```python
from build123d import *

# Parameters (mm, degrees)
BOSS_EXTRUDE1_DEPTH = 84.666666667
SKETCH2_R           = 53.34
CUT_EXTRUDE1_DEPTH  = 85.666666667
SKETCH3_W           = 25.4
SKETCH3_H           = 25.4
BOSS_EXTRUDE2_DEPTH = 44.45
SKETCH5_R           = 3.175
CUT_EXTRUDE2_DEPTH  = 70.215


with BuildPart() as part:
    # Sketch1 → Boss-Extrude1 (new body)
    with BuildSketch(Plane.XY):
        with BuildLine():
            Line((-12.7, -56.515), (12.7, -56.515))
            Line((12.7, -56.515), (12.7, -55.069548981))
            ThreePointArc((12.7, -55.069548981), (0, 56.515), (-12.7, -55.069548981))
            Line((-12.7, -55.069548981), (-12.7, -56.515))
        make_face()
    extrude(amount=BOSS_EXTRUDE1_DEPTH)

    # Sketch2 → Cut-Extrude1 (cut, through all)
    with BuildSketch(Plane.XY.offset(84.666666667)):
        Circle(SKETCH2_R)
    extrude(amount=-CUT_EXTRUDE1_DEPTH, mode=Mode.SUBTRACT)

    # Sketch3 → Boss-Extrude2 (add)
    with BuildSketch(Plane.XZ.offset(56.515)):
        with Locations((0, 42.333333333)):
            Rectangle(SKETCH3_W, SKETCH3_H)
    extrude(amount=BOSS_EXTRUDE2_DEPTH)

    # Sketch5 → Cut-Extrude2 (cut, through all)
    with BuildSketch(Plane(origin=(12.7, 0, 0), x_dir=(0, 0, -1), z_dir=(1, 0, 0))):
        with Locations((-42.333333333, -75.565)):
            Circle(SKETCH5_R)
    extrude(amount=-CUT_EXTRUDE2_DEPTH, mode=Mode.SUBTRACT)


solid = part.part
```
For this review, take the finished solid that the model builds, in its own axes (mm). A direction names the side the tool comes from. Coordinates: 2 decimals unless noted, no trailing zeros. Write each loop counter-clockwise with the first axis right and the second up, starting at its lowest first coordinate (ties: lowest second). Pieces come first, ordered by that corner, then holes.
(1) Add section C-C on x = 0. Give the boundary of the cut face in (y, z) (3 decimals).
(2) Tool access review of faces 1 (the face through (0, -56.515, 15)), 2 (the face through (-12.7, -73, 45)), 3 (the face through (12.7, -78, 45)), 4 (the face through (0, -78, 55.033)): name each direction out of +Z, -Z, +X, -X, +Y, -Y from which nothing blocks a thin tool from reaching the whole face with its end or side.
(3) Add section A-A on y = 0. Give the boundary of the cut face in (x, z) (3 decimals).
(4) The part is to be moulded in two halves that separate along Y. For faces 5 (the face through (0.178, -75.425, 45.505)), 6 (the face through (-6.944, 52.886, 42.926)), 7 (the face through (0, -78, 29.633)), 8 (the face through (0, -56.515, 70)), say which applies: +Y half, -Y half, draft (parallel to the pull), parting line (faces both ways), or undercut.
(5) Wall thickness on probe 1 along Y at (x, z) = (0, 42) (3 decimals); probe 2 along Y at (x, z) = (-2, 21) (1 decimal); probe 3 along X at (y, z) = (-1, 15.5): over which ranges is each line inside the solid? List them lowest first.
(6) For pin 1 Ø23 at (y, z) = (-68.5, 40.5) entering from +X; pin 2 Ø7.5 at (x, y) = (4.5, -83) entering from -Z; pin 3 Ø20.5 at (x, z) = (3.5, 71) entering from -Y (3 decimals), all flat-tipped, find the tip position at first contact; note any pin that passes through.
(7) Add section D-D on x = 28.5. Give the boundary of the cut face in (y, z).
(8) Add section B-B on z = 8. Give the boundary of the cut face in (x, y) (3 decimals), then the cut area to 3 significant figures.
Answer sheet:
1. outline: (-100.965, 29.633) - (-56.515, 29.633) - (-56.515, 0) - (-53.34, 0) - (-53.34, 84.667) - (-56.515, 84.667) - (-56.515, 55.033) - (-100.965, 55.033) - close; (53.34, 0) - (56.515, 0) - (56.515, 84.667) - (53.34, 84.667) - close; hole circle Ø6.35 at (-75.565, 42.333)
2. face 1: -Z, +X, -X, -Y
2. face 2: +Z, -Z, -X, -Y
2. face 3: +Z, -Z, +X, -Y
2. face 4: +Z, +X, -X, -Y
3. outline: (-56.515, 0) - (-53.34, 0) - (-53.34, 84.667) - (-56.515, 84.667) - close; (53.34, 0) - (56.515, 0) - (56.515, 84.667) - (53.34, 84.667) - close
4. face 5: undercut
4. face 6: undercut
4. face 7: draft
4. face 8: -Y half
5. probe 1: y = -100.965 to -78.722, -72.408 to -53.34, 53.34 to 56.515
5. probe 2: y = -56.5 to -53.3, 53.3 to 56.5
5. probe 3: x = -56.51 to -53.33, 53.33 to 56.51
6. pin 1: stops at x = 12.7
6. pin 2: stops at z = 29.63
6. pin 3: stops at y = -56.515
7. outline: (-48.8, 0) - (-45.09, 0) - (-45.09, 84.67) - (-48.8, 84.67) - close; (45.09, 0) - (48.8, 0) - (48.8, 84.67) - (45.09, 84.67) - close
8. outline: (-12.7, -56.515) - (12.7, -56.515) - (12.7, -55.07) arc R56.515 ccw (long way) to (-12.7, -55.07) - close; hole circle Ø106.68 at (0, 0)
8. area: 1,110 mm2
